Verification items for the finished model (mm, model axes). A direction names the side the tool comes from. Round coordinates to 2 decimals unless told otherwise and drop trailing zeros. Write each loop counter-clockwise with the first axis right and the second up, starting at its lowest first coordinate (ties: lowest second). Pieces come first, ordered by that corner, then holes. Notation, with made-up numbers: M 4.25,-2 L 57.25,-2 A7 cw 57.25,8 Z; hole C -32.5,49 d11. An arc over 180 degrees is marked long. One line per question, with ' | ' between items.
from build123d import *

# Parameters (mm, degrees)
SKETCH_1_R                  = 1.55
SKETCH_1_R_2                = 3
SKETCH_1_R_3                = 1.05
SKETCH_1_R_4                = 7.5
SKETCH_1_R_5                = 6.5
SKETCH_1_R_6                = 2.85
SKETCH_1_W                  = 5
SKETCH_1_H                  = 8
SKETCH_1_W_2                = 6.1
SKETCH_1_H_2                = 15.1
SKETCH_1_W_3                = 8
SKETCH_1_H_3                = 3.1
EXTRUDE_1_DEPTH             = 3
HOLE_WIZARD_M3_1_AT_2_COUNT = 2
HOLE_WIZARD_M3_1_AT_2_PITCH = 16
FILLET_1_R                  = 5
SKETCH_5_R                  = 1.05
CUT_EXTRUDE_1_DEPTH         = 10
SKETCH_7_R                  = 1.05
CUT_EXTRUDE_3_DEPTH         = 107.88064605


# Read off the part's stored shape, not the designer's step: M3 六角凹锥坑螺钉的锥形沉头孔2
with BuildPart() as part:
    # 草图1 → 凸台-拉伸1 (new body)
    with BuildSketch(Plane.XY):
        with BuildLine():
            Line((57.45, 12), (57.45, -12))
            Line((57.45, -12), (57.45, -17.45))
            Line((57.45, -17.45), (69, -17.45))
            Line((69, -17.45), (69, -30.45))
            Line((69, -30.45), (94.15, -30.45))
            Line((94.15, -30.45), (94.15, -40.55))
            Line((94.15, -40.55), (69, -40.55))
            Line((69, -40.55), (54.9, -40.55))
            Line((54.9, -40.55), (51.85, -37.5))
            Line((51.85, -37.5), (33.823069051, -37.5))
            ThreePointArc((33.823069051, -37.5), (0, -50.5), (-33.823069051, -37.5))
            Line((-33.823069051, -37.5), (-51.85, -37.5))
            Line((-51.85, -37.5), (-57.45, -37.5))
            Line((-57.45, -37.5), (-57.45, -17.45))
            Line((-57.45, -17.45), (-57.45, 17.45))
            Line((-57.45, 17.45), (-57.45, 37.5))
            Line((-57.45, 37.5), (-51.85, 37.5))
            Line((-51.85, 37.5), (-33.823069051, 37.5))
            ThreePointArc((-33.823069051, 37.5), (-4.723449629, 50.278613979), (26.246992614, 43.143312097))
            Line((26.246992614, 43.143312097), (39.651749171, 43.143312097))
            Line((39.651749171, 43.143312097), (39.651749171, 31.470777261))
            Line((39.651749171, 31.470777261), (57.45, 12))
        make_face()
        with Locations((-53.45, 24.5)):
            Circle(SKETCH_1_R, mode=Mode.SUBTRACT)
        with Locations((-53.45, -24.5)):
            Circle(SKETCH_1_R, mode=Mode.SUBTRACT)
        with Locations((-20.45, 8)):
            Circle(SKETCH_1_R, mode=Mode.SUBTRACT)
        with Locations((-20.45, -8)):
            Circle(SKETCH_1_R, mode=Mode.SUBTRACT)
        with Locations(Location((20.45, -8, 0), (0, 0, 180))):
            Circle(SKETCH_1_R, mode=Mode.SUBTRACT)
        with Locations(Location((20.45, 8, 0), (0, 0, 180))):
            Circle(SKETCH_1_R, mode=Mode.SUBTRACT)
        with Locations((53.45, 8)):
            Circle(SKETCH_1_R, mode=Mode.SUBTRACT)
        with Locations((53.45, -8)):
            Circle(SKETCH_1_R, mode=Mode.SUBTRACT)
        with Locations((-46.5, 0)):
            Circle(SKETCH_1_R, mode=Mode.SUBTRACT)
        with Locations((-24.984431788, 39.21770223)):
            Circle(SKETCH_1_R, mode=Mode.SUBTRACT)
        with Locations((19.651749171, 42.143312097)):
            Circle(SKETCH_1_R, mode=Mode.SUBTRACT)
        with Locations(Location((19.651749171, -42.143312097, 0), (0, 0, 180))):
            Circle(SKETCH_1_R, mode=Mode.SUBTRACT)
        with Locations(Location((-24.984431788, -39.21770223, 0), (0, 0, 180))):
            Circle(SKETCH_1_R, mode=Mode.SUBTRACT)
        with Locations((-10.715136106, 25.86862691)):
            Circle(SKETCH_1_R, mode=Mode.SUBTRACT)
        with Locations((10.715136106, 25.86862691)):
            Circle(SKETCH_1_R, mode=Mode.SUBTRACT)
        with Locations((25.86862691, 10.715136106)):
            Circle(SKETCH_1_R, mode=Mode.SUBTRACT)
        with Locations((25.86862691, -10.715136106)):
            Circle(SKETCH_1_R, mode=Mode.SUBTRACT)
        with Locations((10.715136106, -25.86862691)):
            Circle(SKETCH_1_R, mode=Mode.SUBTRACT)
        with Locations((-10.715136106, -25.86862691)):
            Circle(SKETCH_1_R, mode=Mode.SUBTRACT)
        with Locations((-25.86862691, -10.715136106)):
            Circle(SKETCH_1_R, mode=Mode.SUBTRACT)
        with Locations((-25.86862691, 10.715136106)):
            Circle(SKETCH_1_R, mode=Mode.SUBTRACT)
        with Locations((-36.95, 15.3)):
            Circle(SKETCH_1_R, mode=Mode.SUBTRACT)
        with Locations((-36.95, -15.3)):
            Circle(SKETCH_1_R, mode=Mode.SUBTRACT)
        with Locations(Location((36.95, -15.3, 0), (0, 0, 180))):
            Circle(SKETCH_1_R, mode=Mode.SUBTRACT)
        with Locations(Location((36.95, 15.3, 0), (0, 0, 180))):
            Circle(SKETCH_1_R, mode=Mode.SUBTRACT)
        with Locations((-15.307337295, 36.9551813)):
            Circle(SKETCH_1_R_2, mode=Mode.SUBTRACT)
        with Locations(Location((15.307337295, 36.9551813, 0), (0, 0, 180))):
            Circle(SKETCH_1_R_2, mode=Mode.SUBTRACT)
        with Locations(Location((-15.307337295, -36.9551813, 0), (0, 0, 180))):
            Circle(SKETCH_1_R_2, mode=Mode.SUBTRACT)
        with Locations((15.307337295, -36.9551813)):
            Circle(SKETCH_1_R_2, mode=Mode.SUBTRACT)
        with Locations((33.03932053, 40.800162976)):
            Circle(SKETCH_1_R_3, mode=Mode.SUBTRACT)
        with Locations((37.123106012, 37.123106012)):
            Circle(SKETCH_1_R_3, mode=Mode.SUBTRACT)
        with Locations((40, 0)):
            Circle(SKETCH_1_R_4, mode=Mode.SUBTRACT)
        with Locations((0, 40)):
            Circle(SKETCH_1_R_5, mode=Mode.SUBTRACT)
        with Locations(Location((0, -40, 0), (0, 0, 180))):
            Circle(SKETCH_1_R_5, mode=Mode.SUBTRACT)
        with Locations(Location((-53.45, -8, 0), (0, 0, 180))):
            Circle(SKETCH_1_R, mode=Mode.SUBTRACT)
        with Locations(Location((-53.45, 8, 0), (0, 0, 180))):
            Circle(SKETCH_1_R, mode=Mode.SUBTRACT)
        with Locations((-20.45, -24.5)):
            Circle(SKETCH_1_R_6, mode=Mode.SUBTRACT)
        with Locations(Location((-20.45, 24.5, 0), (0, 0, 180))):
            Circle(SKETCH_1_R_6, mode=Mode.SUBTRACT)
        with Locations(Location((53.45, -24.5, 0), (0, 0, 180))):
            Circle(SKETCH_1_R, mode=Mode.SUBTRACT)
        with Locations((-34, 0)):
            Circle(SKETCH_1_R_4, mode=Mode.SUBTRACT)
        with BuildLine():
            Line((-17.45, 18.594286757), (-17.45, -18.594286757))
            ThreePointArc((-17.45, -18.594286757), (0, -25.5), (17.45, -18.594286757))
            Line((17.45, -18.594286757), (17.45, 18.594286757))
            ThreePointArc((17.45, 18.594286757), (0, 25.5), (-17.45, 18.594286757))
        make_face(mode=Mode.SUBTRACT)
        with Locations((-26.95, -29.5)):
            Rectangle(SKETCH_1_W, SKETCH_1_H, mode=Mode.SUBTRACT)
        with Locations((-46.95, 29.5)):
            Rectangle(SKETCH_1_W, SKETCH_1_H, mode=Mode.SUBTRACT)
        with Locations((-46.95, -29.5)):
            Rectangle(SKETCH_1_W, SKETCH_1_H, mode=Mode.SUBTRACT)
        with Locations((-26.95, 29.5)):
            Rectangle(SKETCH_1_W, SKETCH_1_H, mode=Mode.SUBTRACT)
        with Locations((46.95, -29.5)):
            Rectangle(SKETCH_1_W, SKETCH_1_H, mode=Mode.SUBTRACT)
        with Locations((26.95, -29.5)):
            Rectangle(SKETCH_1_W, SKETCH_1_H, mode=Mode.SUBTRACT)
        with Locations((26.95, 29.5)):
            Rectangle(SKETCH_1_W, SKETCH_1_H, mode=Mode.SUBTRACT)
        with Locations((61.95, -29)):
            Rectangle(SKETCH_1_W_2, SKETCH_1_H_2, mode=Mode.SUBTRACT)
        with Locations((86.95, -36)):
            Rectangle(SKETCH_1_W_3, SKETCH_1_H_3, mode=Mode.SUBTRACT)
    extrude(amount=EXTRUDE_1_DEPTH)

    # 草图3 → M3 六角凹锥坑螺钉的锥形沉头孔1 (revolve, cut)
    with BuildSketch(Plane(origin=(-53.45, -8, 3), x_dir=(0, -1, 0), z_dir=(1, 0, 0))):
        Polygon((0, 0), (0, 3), (1.5, 3), (1.5, 1.86), (3.36, 0), align=None)
    hole_wizard_m3_1 = revolve(axis=Axis((-53.45, -8, 9.35), (0, 0, -1)), mode=Mode.SUBTRACT)

    # M3 六角凹锥坑螺钉的锥形沉头孔1 at 2: M3 六角凹锥坑螺钉的锥形沉头孔1 ×2
    with Locations(*[(0, i * HOLE_WIZARD_M3_1_AT_2_PITCH, 0) for i in range(1, HOLE_WIZARD_M3_1_AT_2_COUNT)]):
        add(hole_wizard_m3_1, mode=Mode.SUBTRACT)

    # 圆角1
    fillet_1_edges = [part.edges().sort_by_distance(p)[0] for p in [
        (17.45, 18.594286757, 1.5),
        (-17.45, 18.594286757, 1.5),
        (-17.45, -18.594286757, 1.5),
        (17.45, -18.594286757, 1.5),
    ]]
    fillet(fillet_1_edges, radius=FILLET_1_R)

    # M3 六角凹锥坑螺钉的锥形沉头孔2 outline → M3 六角凹锥坑螺钉的锥形沉头孔2 (revolve, cut)
    with BuildSketch(Plane(origin=(53.45, 8, 0), x_dir=(1, 0, 0), z_dir=(0, -1, 0))):
        Polygon((1.55, 3), (1.55, 1.19), (3.36, 3), align=None)
    revolve(axis=Axis((53.45, 8, 0), (0, 0, 1)), mode=Mode.SUBTRACT)

    # Hole Wizard M3 _2 2 outline → Hole Wizard M3 _2 2 (revolve, cut)
    with BuildSketch(Plane(origin=(53.45, -8, 0), x_dir=(1, 0, 0), z_dir=(0, -1, 0))):
        Polygon((1.55, 3), (1.55, 1.19), (3.36, 3), align=None)
    revolve(axis=Axis((53.45, -8, 0), (0, 0, 1)), mode=Mode.SUBTRACT)

    # Hole Wizard M3 _2 3 outline → Hole Wizard M3 _2 3 (revolve, cut)
    with BuildSketch(Plane(origin=(53.45, -24.5, 0), x_dir=(1, 0, 0), z_dir=(0, -1, 0))):
        Polygon((1.55, 3), (1.55, 1.19), (3.36, 3), align=None)
    revolve(axis=Axis((53.45, -24.5, 0), (0, 0, 1)), mode=Mode.SUBTRACT)

    # Hole Wizard M3 _2 4 outline → Hole Wizard M3 _2 4 (revolve, cut)
    with BuildSketch(Plane(origin=(-36.95, 15.3, 0), x_dir=(1, 0, 0), z_dir=(0, -1, 0))):
        Polygon((1.55, 3), (1.55, 1.19), (3.36, 3), align=None)
    revolve(axis=Axis((-36.95, 15.3, 0), (0, 0, 1)), mode=Mode.SUBTRACT)

    # Hole Wizard M3 _2 5 outline → Hole Wizard M3 _2 5 (revolve, cut)
    with BuildSketch(Plane(origin=(-36.95, -15.3, 0), x_dir=(1, 0, 0), z_dir=(0, -1, 0))):
        Polygon((1.55, 3), (1.55, 1.19), (3.36, 3), align=None)
    revolve(axis=Axis((-36.95, -15.3, 0), (0, 0, 1)), mode=Mode.SUBTRACT)

    # Hole Wizard M3 _2 6 outline → Hole Wizard M3 _2 6 (revolve, cut)
    with BuildSketch(Plane(origin=(36.95, 15.3, 0), x_dir=(1, 0, 0), z_dir=(0, -1, 0))):
        Polygon((1.55, 3), (1.55, 1.19), (3.36, 3), align=None)
    revolve(axis=Axis((36.95, 15.3, 0), (0, 0, 1)), mode=Mode.SUBTRACT)

    # Hole Wizard M3 _2 7 outline → Hole Wizard M3 _2 7 (revolve, cut)
    with BuildSketch(Plane(origin=(36.95, -15.3, 0), x_dir=(1, 0, 0), z_dir=(0, -1, 0))):
        Polygon((1.55, 3), (1.55, 1.19), (3.36, 3), align=None)
    revolve(axis=Axis((36.95, -15.3, 0), (0, 0, 1)), mode=Mode.SUBTRACT)

    # Hole Wizard M3 _2 8 outline → Hole Wizard M3 _2 8 (revolve, cut)
    with BuildSketch(Plane(origin=(25.86862691, 10.715136106, 0), x_dir=(1, 0, 0), z_dir=(0, -1, 0))):
        Polygon((3.36, 0), (1.55, 1.81), (1.55, 0), align=None)
    revolve(axis=Axis((25.86862691, 10.715136106, 0), (0, 0, 1)), mode=Mode.SUBTRACT)

    # Hole Wizard M3 _2 9 outline → Hole Wizard M3 _2 9 (revolve, cut)
    with BuildSketch(Plane(origin=(25.86862691, -10.715136106, 0), x_dir=(1, 0, 0), z_dir=(0, -1, 0))):
        Polygon((3.36, 0), (1.55, 1.81), (1.55, 0), align=None)
    revolve(axis=Axis((25.86862691, -10.715136106, 0), (0, 0, 1)), mode=Mode.SUBTRACT)

    # Hole Wizard M3 _2 10 outline → Hole Wizard M3 _2 10 (revolve, cut)
    with BuildSketch(Plane(origin=(-25.86862691, 10.715136106, 0), x_dir=(1, 0, 0), z_dir=(0, -1, 0))):
        Polygon((3.36, 0), (1.55, 1.81), (1.55, 0), align=None)
    revolve(axis=Axis((-25.86862691, 10.715136106, 0), (0, 0, 1)), mode=Mode.SUBTRACT)

    # Hole Wizard M3 _2 11 outline → Hole Wizard M3 _2 11 (revolve, cut)
    with BuildSketch(Plane(origin=(-25.86862691, -10.715136106, 0), x_dir=(1, 0, 0), z_dir=(0, -1, 0))):
        Polygon((3.36, 0), (1.55, 1.81), (1.55, 0), align=None)
    revolve(axis=Axis((-25.86862691, -10.715136106, 0), (0, 0, 1)), mode=Mode.SUBTRACT)

    # 草图5 → 切除-拉伸1 (cut)
    with BuildSketch(Plane(origin=(0, 0, 0), x_dir=(-1, 0, 0), z_dir=(0, 0, -1))):
        with Locations((-65, -35.5)):
            Circle(SKETCH_5_R)
        with Locations((-58.9, -35.5)):
            Circle(SKETCH_5_R)
        with Locations((-65, -22.5)):
            Circle(SKETCH_5_R)
        with Locations((-58.9, -22.5)):
            Circle(SKETCH_5_R)
    extrude(amount=-CUT_EXTRUDE_1_DEPTH, mode=Mode.SUBTRACT)

    # 草图7 → 切除-拉伸3 (cut, through all)
    with BuildSketch(Plane(origin=(0, 0, 0), x_dir=(-1, 0, 0), z_dir=(0, 0, -1))):
        with Locations((-89.9, -37.55)):
            Circle(SKETCH_7_R)
        with Locations((-89.9, -34.45)):
            Circle(SKETCH_7_R)
        with Locations((-84, -34.45)):
            Circle(SKETCH_7_R)
        with Locations((-84, -37.55)):
            Circle(SKETCH_7_R)
        with Locations((84, -37.55)):
            Circle(SKETCH_7_R)
        with Locations((84, -34.45)):
            Circle(SKETCH_7_R)
        with Locations((89.9, -34.45)):
            Circle(SKETCH_7_R)
        with Locations((89.9, -37.55)):
            Circle(SKETCH_7_R)
    extrude(amount=-CUT_EXTRUDE_3_DEPTH, mode=Mode.SUBTRACT)


solid = part.part
1. Go/stop test with flat-tipped pins: P1, Ø1.5, axis at x = 41, z = 2, coming from the -Y side; P2, Ø1, axis at y = -26.5, z = 1.5, coming from the +X side; P3, Ø1.5, axis at y = 28, z = 2, coming from the +X side. Record where each tip stops, or that it passes through.
Results:
P1: stops at y = -37.5 | P2: stops at x = 69 | P3: stops at x = 43.51
2. Section check A-A, the plane x = 46. Record the cut outline in (y, z).
Results:
outline: M -37.5,0 L -33.5,0 L -33.5,3 L -37.5,3 Z; M -25.5,0 L -4.5,0 L -4.5,3 L -25.5,3 Z; M 4.5,0 L 24.53,0 L 24.53,3 L 4.5,3 Z
3. Mould release check, pull along Y, two halves, no side actions. Record for faces 4 (the face through (-46, 37.5, 1)), 5 (the face through (94.15, -35, 1)), 6 (the face through (13.69, 34.43, 1.48)), 7 (the face through (-24.45, -30, 1)): pulls with the +Y half, pulls with the -Y half, needs draft (parallel to the pull), parting line crosses it, or undercut.
Results:
face 4: pulls with the +Y half | face 5: needs draft | face 6: undercut | face 7: undercut
4. Thickness scan on line 1 (Y direction, x = -0.5, z = 1.55); line 2 (X direction, y = -2, z = 2); line 3 (Y direction, x = 63.5, z = 2.55). Record the ranges inside material, lowest first.
Results:
line 1: y = -50.5 to -46.48, -33.52 to -25.5, 25.5 to 33.52, 46.48 to 50.5 | line 2: x = -57.45 to -41.23, -26.77 to -17.45, 17.45 to 32.77, 47.23 to 57.45 | line 3: y = -40.55 to -36.55, -21.45 to -17.45
5. Section check B-B, the plane z = 0.5. Count the separate pieces of the cut face and the enclosed holes in it, then the cut area to 3 significant figures.
Results:
separate pieces: 1 | enclosed holes: 50 | area: 7,020 mm2
6. Tool access check on faces 1 (the face through (-49.45, -30, 1)), 2 (the face through (63, -17.45, 1)), 3 (the face through (0.519, -50.497, 1.479)). Record the directions out of +Z, -Z, +X, -X, +Y, -Y that give a thin tool (end or side, any length) a straight path to the whole face; none if there is none.
Results:
face 1: +Z, -Z | face 2: +Z, -Z, +X, +Y | face 3: +Z, -Z, -Y
